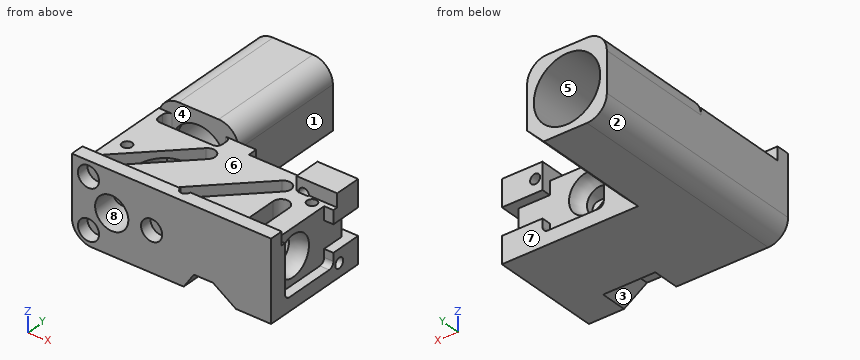
```python
from build123d import *

# Parameters (mm, degrees)
SKETCH1_W                        = 15
SKETCH1_H                        = 6
MAIN_BODY_EXT_DEPTH              = 8.3
EMISSION_PATH_EXT_DEPTH          = 9
SKETCH3_R                        = 1.25
EMISSION_AND_GRIN_CUT_DEPTH      = 20.092931
SKETCH4_R                        = 1
DRUM_LENS_CUT_DEPTH              = 13
SKETCH41_R                       = 1
ADDTL_LIGHT_SOURCE_DEPTH         = 5
SKETCH5_W                        = 15
SKETCH5_H                        = 7.3
FILTERCOVER_CUT1_DEPTH           = 1
TOP_LED_SCREW_W                  = 3.06
TOP_LED_SCREW_H                  = 2
BOSS_EXTRUDE1_DEPTH              = 1
FILTERSET_CUT2_DEPTH             = 4
SKETCH10_R                       = 2.5
EMISSION_LENS_CUT_DEPTH          = 8.5
SKETCH15_R                       = 0.795
MAGNETS_CUT_DEPTH                = 0.9
SCREW_HOLES_CUT_DEPTH            = 20.507434
SCREW_HOLES_CUT_DEPTH_BACK       = 2.5
SKETCH18_R                       = 0.375
EXTERNAL_FILLET_1_R              = 1.5
VERTICAL_PATH_CUT_DEPTH          = 14.011149
VERTICAL_PATH_CUT_DEPTH_BACK     = 4
SKETCH28_R                       = 1.5
CUT_EXTRUDE_ORIGINAL_LIGHT_DEPTH = 0.7
CUT_EXTRUDE_ADDTL_LIGHT_DEPTH    = 0.7
SKETCH29_R                       = 0.375
SIDE_LED_SCREW_DEPTH             = 2.5
SKETCH32_W                       = 2
SKETCH32_H                       = 2.36
SIDE_WIRE_SLOT_CUT_DEPTH         = 0.7
SKETCH45_W                       = 2.36
SKETCH45_H                       = 2
TOP_LED_SLOT_DEPTH               = 0.7
CUT_EXTRUDE16_DEPTH              = 9
CUT_EXTRUDE17_REACH              = 13.945
SKETCH37_R                       = 2
SKETCH51_R                       = 0.375
TOP_LE_SCREW_DEPTH               = 2.1
NOTCH_EXTRUDE_DEPTH              = 2


with BuildPart() as part:
    # Sketch1 → Main Body Ext (new body)
    with BuildSketch(Plane(origin=(0, 0, 0), x_dir=(1, 0, 0), z_dir=(0, 1, 0))):
        Rectangle(SKETCH1_W, SKETCH1_H)
    extrude(amount=MAIN_BODY_EXT_DEPTH)

    # Sketch8 → Emission Path Ext (add)
    with BuildSketch(Plane(origin=(0, 8.3, 0), x_dir=(1, 0, 0), z_dir=(0, 1, 0))):
        Polygon((-2.75, 3), (-1.5, 1.75), (-1.5, -3), (-7.5, -3), (-7.5, 3), align=None)
    extrude(amount=EMISSION_PATH_EXT_DEPTH)

    # Sketch3 → Emission and Grin Cut (cut, through all)
    with BuildSketch(Plane.XZ):
        with Locations(Location((-4.5, 0, 0), (0, 0, 270))):
            Circle(SKETCH3_R)
    extrude(amount=-EMISSION_AND_GRIN_CUT_DEPTH, mode=Mode.SUBTRACT)

    # Sketch4 → Drum Lens Cut (cut)
    with BuildSketch(Plane(origin=(7.5, 0, 0), x_dir=(0, 0, -1), z_dir=(1, 0, 0))):
        with Locations((0, 3)):
            Circle(SKETCH4_R)
    extrude(amount=-DRUM_LENS_CUT_DEPTH, mode=Mode.SUBTRACT)

    # Sketch41 → Addtl Light Source (cut)
    with BuildSketch(Plane(origin=(0, 8.3, 0), x_dir=(1, 0, 0), z_dir=(0, 1, 0))):
        with Locations(Location((1.5, 0, 0), (0, 0, 270))):
            Circle(SKETCH41_R)
    extrude(amount=-ADDTL_LIGHT_SOURCE_DEPTH, mode=Mode.SUBTRACT)

    # Sketch5 → FilterCover Cut1 (cut)
    with BuildSketch(Plane.XY.offset(3)):
        with Locations((0, 4.65)):
            Rectangle(SKETCH5_W, SKETCH5_H)
    extrude(amount=-FILTERCOVER_CUT1_DEPTH, mode=Mode.SUBTRACT)

    # Top-LED-Screw → Boss-Extrude1 (add)
    with BuildSketch(Plane.XY.offset(2)):
        with Locations((5.97, 7.3)):
            Rectangle(TOP_LED_SCREW_W, TOP_LED_SCREW_H)
    extrude(amount=BOSS_EXTRUDE1_DEPTH)

    # Sketch6 → FilterSet Cut2 (cut)
    with BuildSketch(Plane.XY.offset(2)):
        with BuildLine():
            Line((5.3, 4.5), (5.3, 1.8))
            ThreePointArc((5.3, 1.8), (5.7, 1.4), (5.3, 1))
            Line((5.3, 1), (4.1, 1))
            ThreePointArc((4.1, 1), (3.7, 1.4), (4.1, 1.8))
            Line((4.1, 1.8), (4.1, 4.5))
            ThreePointArc((4.1, 4.5), (4.7, 5.1), (5.3, 4.5))
        make_face()
        with BuildLine():
            Line((-6.9, 7.9), (-6.9, 7.5))
            ThreePointArc((-6.9, 7.5), (-6.782843, 7.217157), (-6.5, 7.1))
            Line((-6.5, 7.1), (-2.5, 7.1))
            ThreePointArc((-2.5, 7.1), (-2.217157, 7.217157), (-2.1, 7.5))
            Line((-2.1, 7.5), (-2.1, 7.9))
            ThreePointArc((-2.1, 7.9), (-2.217157, 8.182843), (-2.5, 8.3))
            Line((-2.5, 8.3), (-6.5, 8.3))
            ThreePointArc((-6.5, 8.3), (-6.782843, 8.182843), (-6.9, 7.9))
        make_face()
        with BuildLine():
            Line((-2.605887, 6.591169), (-6.848528, 2.348528))
            ThreePointArc((-6.848528, 2.348528), (-6.848528, 1.5), (-6, 1.5))
            Line((-6, 1.5), (-1.757359, 5.742641))
            ThreePointArc((-1.757359, 5.742641), (-1.757359, 6.591169), (-2.605887, 6.591169))
        make_face()
        with BuildLine():
            Line((3.112092, 6.591169), (-1.130548, 2.348528))
            ThreePointArc((-1.130548, 2.348528), (-1.130548, 1.5), (-0.28202, 1.5))
            Line((-0.28202, 1.5), (3.96062, 5.742641))
            ThreePointArc((3.96062, 5.742641), (3.96062, 6.591169), (3.112092, 6.591169))
        make_face()
    extrude(amount=-FILTERSET_CUT2_DEPTH, mode=Mode.SUBTRACT)

    # Sketch10 → Emission Lens Cut (cut)
    with BuildSketch(Plane(origin=(0, 17.3, 0), x_dir=(1, 0, 0), z_dir=(0, 1, 0))):
        with Locations(Location((-4.5, 0, 0), (0, 0, 270))):
            Circle(SKETCH10_R)
    extrude(amount=-EMISSION_LENS_CUT_DEPTH, mode=Mode.SUBTRACT)

    # Sketch15 → Magnets Cut (cut)
    with BuildSketch(Plane.XZ):
        with Locations(Location((-6.25, -1.875, 0), (0, 0, 270))):
            Circle(SKETCH15_R)
        with Locations(Location((-6.25, 1.875, 0), (0, 0, 270))):
            Circle(SKETCH15_R)
        with Locations(Location((-1.5, 0, 0), (0, 0, 270))):
            Circle(SKETCH15_R)
    extrude(amount=-MAGNETS_CUT_DEPTH, mode=Mode.SUBTRACT)

    # Sketch18 → Screw Holes Cut (cut, two sides: drawn at the far end of the back side and taken through both)
    with BuildSketch(Plane.XY.offset(2).offset(-SCREW_HOLES_CUT_DEPTH_BACK)):
        with Locations(Location((-6.5, 4, 0), (0, 0, 180))):
            Circle(SKETCH18_R)
        with Locations(Location((6, 5.8, 0), (0, 0, 180))):
            Circle(SKETCH18_R)
        with Locations((0.25, 1)):
            Circle(SKETCH18_R)
    extrude(amount=SCREW_HOLES_CUT_DEPTH + SCREW_HOLES_CUT_DEPTH_BACK, mode=Mode.SUBTRACT)

    # External Fillet 1
    # the kernel refuses this fillet: 1.5 mm, written as the material it takes off along each edge
    with BuildSketch(Plane(origin=(-7.5, -3.75, -3), x_dir=(1, 0, 0), z_dir=(0, 1, 0))) as external_fillet_1_piece_1:
        with BuildLine():
            CenterArc((EXTERNAL_FILLET_1_R, -EXTERNAL_FILLET_1_R), EXTERNAL_FILLET_1_R, 90, 90)
            Line((0, -EXTERNAL_FILLET_1_R), (0, 0))
            Line((0, 0), (EXTERNAL_FILLET_1_R, 0))
        make_face()
    extrude(amount=24.8, mode=Mode.SUBTRACT)
    with BuildSketch(Plane(origin=(-1.5, 8.3, 3), x_dir=(0, 0, -1), z_dir=(0, 1, 0))) as external_fillet_1_piece_2:
        with BuildLine():
            CenterArc((EXTERNAL_FILLET_1_R, EXTERNAL_FILLET_1_R), EXTERNAL_FILLET_1_R, 180, 90)
            Line((0, EXTERNAL_FILLET_1_R), (0, 0))
            Line((0, 0), (EXTERNAL_FILLET_1_R, 0))
        make_face()
    extrude(amount=12.75, mode=Mode.SUBTRACT)

    # Sketch28 → Vertical-Path-Cut (cut, two sides: drawn at the far end of the back side and taken through both)
    with BuildSketch(Plane(origin=(0, 7.1, 0), x_dir=(1, 0, 0), z_dir=(0, 1, 0)).offset(-VERTICAL_PATH_CUT_DEPTH_BACK)):
        with Locations(Location((-4.5, 0, 0), (0, 0, 180))):
            Circle(SKETCH28_R)
    extrude(amount=VERTICAL_PATH_CUT_DEPTH + VERTICAL_PATH_CUT_DEPTH_BACK, mode=Mode.SUBTRACT)

    # Sketch12 → Cut-Extrude Original Light (cut)
    with BuildSketch(Plane(origin=(7.5, 0, 0), x_dir=(0, 0, -1), z_dir=(1, 0, 0))):
        with BuildLine():
            Line((1.6, 5.94), (-1.6, 5.94))
            Line((-1.6, 5.94), (-2, 5.94))
            Line((-2, 5.94), (-2, 1.33))
            Line((-2, 1.33), (1.6, 1.33))
            ThreePointArc((1.6, 1.33), (1.882843, 1.447157), (2, 1.73))
            Line((2, 1.73), (2, 5.54))
            ThreePointArc((2, 5.54), (1.882843, 5.822843), (1.6, 5.94))
        make_face()
    extrude(amount=-CUT_EXTRUDE_ORIGINAL_LIGHT_DEPTH, mode=Mode.SUBTRACT)

    # Sketch44 → Cut-Extrude Addtl Light (cut)
    with BuildSketch(Plane(origin=(0, 8.3, 0), x_dir=(1, 0, 0), z_dir=(0, 1, 0))):
        with BuildLine():
            Line((-0.17, -2), (4.44, -2))
            Line((4.44, -2), (4.44, 1.6))
            ThreePointArc((4.44, 1.6), (4.322843, 1.882843), (4.04, 2))
            Line((4.04, 2), (0.23, 2))
            ThreePointArc((0.23, 2), (-0.052843, 1.882843), (-0.17, 1.6))
            Line((-0.17, 1.6), (-0.17, -2))
        make_face()
    extrude(amount=-CUT_EXTRUDE_ADDTL_LIGHT_DEPTH, mode=Mode.SUBTRACT)

    # Sketch29 → Side-LED-Screw (cut)
    with BuildSketch(Plane(origin=(7.5, 0, 0), x_dir=(0, 0, -1), z_dir=(1, 0, 0))):
        with Locations((2, 6.5)):
            Circle(SKETCH29_R)
    extrude(amount=-SIDE_LED_SCREW_DEPTH, mode=Mode.SUBTRACT)

    # Sketch32 → Side-Wire-Slot-Cut (cut)
    with BuildSketch(Plane(origin=(7.5, 0, 0), x_dir=(0, 0, -1), z_dir=(1, 0, 0))):
        with Locations((0, 7.12)):
            Rectangle(SKETCH32_W, SKETCH32_H)
    extrude(amount=-SIDE_WIRE_SLOT_CUT_DEPTH, mode=Mode.SUBTRACT)

    # Sketch45 → Top-LED-slot (cut)
    with BuildSketch(Plane(origin=(0, 8.3, 0), x_dir=(1, 0, 0), z_dir=(0, 1, 0))):
        with Locations((5.62, 0)):
            Rectangle(SKETCH45_W, SKETCH45_H)
    extrude(amount=-TOP_LED_SLOT_DEPTH, mode=Mode.SUBTRACT)

    # Sketch33 → Side-BallLens_Cut (revolve, cut)
    with BuildSketch(Plane.XY, mode=Mode.PRIVATE) as side_balllens_cut_sk:
        with BuildLine():
            Line((6.8, 3), (5.3, 3))
            ThreePointArc((5.3, 3), (5.73934, 4.06066), (6.8, 4.5))
            Line((6.8, 4.5), (6.8, 3))
        make_face()
    revolve(side_balllens_cut_sk.sketch.rotate(Axis((6.8, 3, 0), (-1, 0, 0)), 84.26086), axis=Axis((6.8, 3, 0), (-1, 0, 0)), mode=Mode.SUBTRACT)

    # Sketch47 → Top-BallLens_Cut (revolve, cut)
    with BuildSketch(Plane(origin=(1.5, 0, 0), x_dir=(0, 0, -1), z_dir=(1, 0, 0))):
        with BuildLine():
            Line((-1.5, 7.6), (0, 7.6))
            Line((0, 7.6), (0, 6.137287))
            ThreePointArc((0, 6.137287), (-1.04756, 6.563498), (-1.5, 7.6))
        make_face()
    revolve(axis=Axis((1.5, 7.6, 0), (0, -1, 0)), mode=Mode.SUBTRACT)

    # Sketch36 → Cut-Extrude16 (cut)
    with BuildSketch(Plane(origin=(0, 17.3, 0), x_dir=(1, 0, 0), z_dir=(0, 1, 0))):
        with BuildLine():
            Line((-7.5, -1.5), (-7.5, -3))
            Line((-7.5, -3), (-6, -3))
            ThreePointArc((-6, -3), (-7.06066, -2.56066), (-7.5, -1.5))
        make_face()
    extrude(amount=-CUT_EXTRUDE16_DEPTH, mode=Mode.SUBTRACT)

    # Sketch37 → Cut-Extrude17 (cut, up to next)
    with BuildSketch(Plane(origin=(0, 8.8, 0), x_dir=(1, 0, 0), z_dir=(0, 1, 0)), mode=Mode.PRIVATE) as cut_extrude17_sk1:
        with Locations(Location((-4.5, 0, 0), (0, 0, 180))):
            Circle(SKETCH37_R)
    cut_extrude17_tool1 = extrude(cut_extrude17_sk1.sketch, amount=-CUT_EXTRUDE17_REACH, mode=Mode.PRIVATE) & part.part
    add(cut_extrude17_tool1.solids().sort_by_distance((-4.5, 8.8, 0))[0], mode=Mode.SUBTRACT)

    # Sketch51 → Top-LE-Screw (cut)
    with BuildSketch(Plane(origin=(0, 8.3, 0), x_dir=(1, 0, 0), z_dir=(0, 1, 0))):
        with Locations(Location((5, -2, 0), (0, 0, 270))):
            Circle(SKETCH51_R)
    extrude(amount=-TOP_LE_SCREW_DEPTH, mode=Mode.SUBTRACT)

    # Notch → Notch-Extrude (cut)
    with BuildSketch(Plane.XZ):
        Polygon((3.12111, -1.8476), (1.684933, -1.8476), (1.684933, -3), (4.84971, -3), align=None)
        Polygon((1.684933, -3), (1.684933, -1.8476), (0.916667, -3), align=None)
    extrude(amount=-NOTCH_EXTRUDE_DEPTH, mode=Mode.SUBTRACT)


solid = part.part
```
Read the model definition and answer for the solid it produces. Units are mm, in the model's axes. Face numbers are marked on the shaded views. A direction names the side the tool comes from. Round coordinates to 2 decimals unless told otherwise and drop trailing zeros. Write each loop counter-clockwise with the first axis right and the second up, starting at its lowest first coordinate (ties: lowest second). Pieces come first, ordered by that corner, then holes. Notation, with made-up numbers: (57, 23.5) - (115, 23.5) arc R22 ccw to (115, 47.5) - close; hole circle Ø10 at (-31.75, 71). An arc over 180 degrees is marked (long way). One line per item, written item: value.
Q1. Which of the six approach directions +Z, -Z, +X, -X, +Y, -Y give full straight-line access (tool end or side, diameter ignored) to the marked faces 1, 2, 3, 4 and 5?
The answers:
face 1: +Z, -Z, +X, +Y
face 2: -Z, -X, +Y, -Y
face 3: -Z, -Y
face 4: +Z
face 5: +Y
Q2. For a pull along Y with two mould halves and no side action, classify the marked faces 6, 7 and 8 as pulls with the +Y half, pulls with the -Y half, needs draft (parallel to the pull), parting line crosses it, or undercut.
The answers:
face 6: undercut
face 7: pulls with the +Y half
face 8: needs draft
Q3. Straight lines are drawn through the part: line 1 (Y direction, x = 0, z = 1); line 2 (Y direction, x = -0.75, z = 0); line 3 (Y direction, x = -4, z = 2.1). For each, find the intervals that lie inside material, in ascending order. Write a range as from..to.
The answers:
line 1: y = 0..0.72, 1.28..1.78, 3.48..7.6
line 2: y = 0.9..1.33, 4..8.3
line 3: y = 0..1, 8.3..8.8
Q4. Find section A-A (y = 16). Determine the outline of the cut face in (x, z), and give its area (3 significant figures).
The answers:
outline: (-7.5, -1.5) arc R1.5 ccw to (-6, -3) - (-2.75, -3) - (-1.5, -1.75) - (-1.5, 1.5) arc R1.5 ccw to (-3, 3) - (-6, 3) arc R1.5 ccw to (-7.5, 1.5) - close; hole circle Ø5 at (-4.5, 0)
area: 14.1 mm2
Q5. Find section B-B (x = -4.75). Count the separate pieces of the cut face and the enclosed holes in it, and give its area (3 significant figures).
The answers:
separate pieces: 4
enclosed holes: 0
area: 26.1 mm2
Q6. This flat-tipped pin is pushed along its axis until it touches: P1, Ø2, axis at x = 6, z = 2.5, coming from the +Y side. Where does it stop, or does it pass through?
The answers:
P1: stops at y = 8.3
